Read the model definition and answer for the solid it produces. Units are mm, in the model's axes. A direction names the side the tool comes from. Round coordinates to 2 decimals unless told otherwise and drop trailing zeros. Order: outer loops, then holes, each group sorted by start corner. A loop starts at its lowest first (then second) coordinate and runs counter-clockwise, first axis right, second up. Notation, with made-up numbers: (65, -33) -> (109, -33) arc R14 cw to (109, -15) -> close; hole circle Ø10 at (-30.75, -34.75). An arc over 180 degrees is marked (long way). One line per item, written item: value. Start each with the question number.
1. Flat-ended cylindrical pins translate along their axes: pin 1 Ø10 at (x, z) = (33.5, -134.5) entering from +Y; pin 2 Ø1.7 at (y, z) = (-0.5, -278.5) entering from +X; pin 3 Ø4 at (y, z) = (1.5, -247) entering from +X. Find the tip coordinate at first contact, or state that the pin passes through.
2. Section A-A (z = -268.5) is taken. Give the vertices of the cut face in (x, y), then the cut area to 3 significant figures.
3. For faces 1 (the face through (1.588, 14, -155)), 2 (the face through (0, 13, -155)), determine the directions among +Z, -Z, +X, -X, +Y, -Y from which every point of the face is accessible in a straight line to the end or side of a thin tool.
4. Section D-D (z = -190.5) is taken. Give the vertices of the cut face in (x, y).
5. Section B-B (x = 64.5) is taken. Give the vertices of the cut face in (y, z), then the cut area to 3 significant figures.
6. Consider line 1 (Y direction, x = 47, z = -291); line 2 (X direction, y = -0.35, z = -31.75); line 3 (X direction, y = 1.75, z = -134). Determine where each line is inside the solid, lowest interval first.
7. Section C-C (y = 21.5) is taken. Give the vertices of the cut face in (x, z), then the cut area to 3 significant figures.
from build123d import *

# Parameters (mm, degrees)
BASE_FLANGE1_DEPTH           = 1.5875
EDGE_FLANGE1_STRIP_W         = 9.5504
EDGE_FLANGE1_STRIP_H         = 1.5875
EDGE_FLANGE1_STRIP_CUT_DEPTH = 304.8
EDGE_FLANGE1_DEPTH           = 304.8
CUT_EXTRUDE1_DEPTH           = 342.722050796
CUT_EXTRUDE1_DEPTH_BACK      = 342.722050796
F_6_CLEARANCE_HOLE1_D        = 3.7973


# Sheet-metal steps are written as plain solids
with BuildPart() as part:
    # Sketch1 → Base-Flange1 (new body)
    with BuildSketch(Plane(origin=(0, 0, 0), x_dir=(1, 0, 0), z_dir=(0, 1, 0))):
        Polygon((0, 304.8), (76.2, 304.8), (152.4, 0), (0, 0), align=None)
    extrude(amount=-BASE_FLANGE1_DEPTH)

    # Edge-Flange1 strip (across the edge) → Edge-Flange1 strip cut (cut)
    with BuildSketch(Plane.XY.offset(-304.8)):
        with Locations((-1.5875, -0.79375)):
            Rectangle(EDGE_FLANGE1_STRIP_W, EDGE_FLANGE1_STRIP_H)
    extrude(amount=EDGE_FLANGE1_STRIP_CUT_DEPTH, mode=Mode.SUBTRACT)

    # Edge-Flange1 section (across the edge) → Edge-Flange1 (add)
    with BuildSketch(Plane.XY.offset(-304.8)):
        with BuildLine():
            Line((0, 1.6002), (0, 25.4))
            Line((0, 25.4), (1.5875, 25.4))
            Line((1.5875, 25.4), (1.5875, 1.6002))
            ThreePointArc((1.5875, 1.6002), (2.056187729, 0.468687729), (3.1877, 0))
            Line((3.1877, 0), (3.1877, -1.5875))
            ThreePointArc((3.1877, -1.5875), (0.933655714, -0.653844286), (0, 1.6002))
        make_face()
    extrude(amount=EDGE_FLANGE1_DEPTH)

    # Sketch10 → Cut-Extrude1 (cut, two sides: drawn at the far end of the back side and taken through both)
    with BuildSketch(Plane(origin=(0, 0, 0), x_dir=(1, 0, 0), z_dir=(0, 1, 0)).offset(-CUT_EXTRUDE1_DEPTH_BACK)):
        Polygon((67.87676626, 967.988947135), (67.87676626, 304.8), (67.87676626, 261.217419128), (67.87676626, 259.06565424), (116.914364331, 113.849879077), (116.914364331, 112.848219234), (117.306905871, 0), (119.613788846, -663.184934911), (1445.325011297, -621.136473854), (1393.587988711, 1010.037408193), align=None)
    extrude(amount=CUT_EXTRUDE1_DEPTH + CUT_EXTRUDE1_DEPTH_BACK, mode=Mode.SUBTRACT)

    # #6 Clearance Hole1 (through all)
    with Locations(Plane(origin=(0, -1.5875, 0), x_dir=(-1, 0, 0), z_dir=(0, -1, 0))):
        with Locations((-55.118000004, 260.349999989), (-104.543184669, 31.750000016), (-104.543184669, 63.500000016)):
            Hole(F_6_CLEARANCE_HOLE1_D / 2)


solid = part.part
Answer:
1. pin 1: y = 0
1. pin 2: x = 67.88
1. pin 3: x = 72.4
2. outline: (0, 1.6) arc R3.19 ccw to (3.19, -1.59) -> (67.88, -1.59) -> (67.88, 0) -> (3.19, 0) arc R1.6 cw to (1.59, 1.6) -> (1.59, 25.4) -> (0, 25.4) -> close
2. area: 146 mm^2
3. face 1: +Z, -Z, +X, +Y
3. face 2: +Z, -Z, -X, +Y, -Y
4. outline: (0, 1.6) arc R3.19 ccw to (3.19, -1.59) -> (91.03, -1.59) -> (91.03, 0) -> (3.19, 0) arc R1.6 cw to (1.59, 1.6) -> (1.59, 25.4) -> (0, 25.4) -> close
5. outline: (-1.59, -304.8) -> (0, -304.8) -> (0, 0) -> (-1.59, 0) -> close
5. area: 484 mm^2
6. line 1: -1.59 to 0
6. line 2: 0.67 to 102.64, 106.44 to 117.2
6. line 3: 0 to 1.59
7. outline: (0, -304.8) -> (1.59, -304.8) -> (1.59, 0) -> (0, 0) -> close
7. area: 484 mm^2
